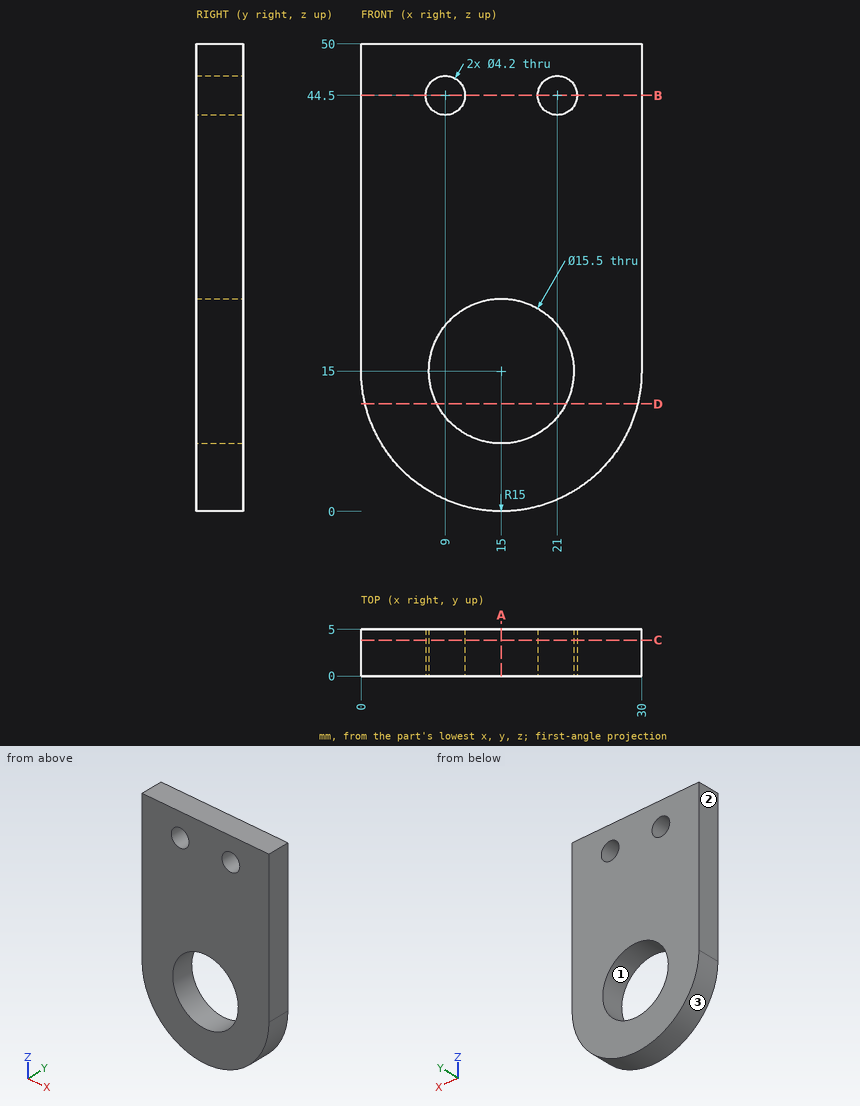
The figure shows three views and two pictorial views of one solid part (mm, origin at its lowest corner). Answer the questions. Coordinates: 2 decimals unless noted, no trailing zeros. Loops run counter-clockwise (first coordinate to the right, second up) from the corner with the lowest first, then second, coordinate; pieces in that order, holes last. Notation, with made-up numbers: (9, -1.5) - (59, -1.5) arc R25 cw to (59, 29.5) - close; hole circle Ø11 at (-39, 9.5). An arc over 180 degrees is marked (long way). Write item = value, one per line.
1) Determine the mould class of the marked faces 1, 2 and 3 for opening direction Z: pulls with the +Z half, pulls with the -Z half, needs draft (parallel to the pull), parting line crosses it, or undercut.
Responses:
face_1 = undercut
face_2 = needs draft
face_3 = pulls with the -Z half
2) Find the intervals of material crossed by line 1 along X through (y, z) = (1.75, 44.5); line 2 along X through (y, z) = (2.35, 15); line 3 along Z through (x, y) = (9.75, 1.9), in increasing order.
Responses:
line_1 = 0 to 6.9, 11.1 to 18.9, 23.1 to 30
line_2 = 0 to 7.25, 22.75 to 30
line_3 = 0.95 to 9.3, 20.7 to 42.54, 46.46 to 50
3) Section A-A (x = 15) is taken. Determine the outline of the cut face in (y, z).
Responses:
outline = (0, 0) - (5, 0) - (5, 7.25) - (0, 7.25) - close; (0, 22.75) - (5, 22.75) - (5, 50) - (0, 50) - close
4) Section B-B (z = 44.5) is taken. Determine the outline of the cut face in (x, y).
Responses:
outline = (0, 0) - (6.9, 0) - (6.9, 5) - (0, 5) - close; (11.1, 0) - (18.9, 0) - (18.9, 5) - (11.1, 5) - close; (23.1, 0) - (30, 0) - (30, 5) - (23.1, 5) - close
5) Section D-D (z = 11.5) is taken. Determine the outline of the cut face in (x, y).
Responses:
outline = (0.41, 0) - (8.09, 0) - (8.09, 5) - (0.41, 5) - close; (21.91, 0) - (29.59, 0) - (29.59, 5) - (21.91, 5) - close
6) Each of these flat-tipped pins is pushed along its axis until it touches: P1, Ø2.5, axis at x = 9, z = 44.5, coming from the +Y side; P2, Ø3, axis at y = 1.5, z = 12.5, coming from the +X side. Where does it stop, or does it pass through?
Responses:
P1 = through
P2 = 29.97
7) Section C-C (y = 3.85) is taken. Determine the outline of the cut face in (x, z).
Responses:
outline = (0, 15) arc R15 ccw to (30, 15) - (30, 50) - (0, 50) - close; hole circle Ø4.2 at (9, 44.5); hole circle Ø15.5 at (15, 15); hole circle Ø4.2 at (21, 44.5)
